```python
from build123d import *

# Parameters (mm, degrees)
CROQUIS1_R              = 5
CROQUIS1_R_2            = 3.25
SALIENTE_EXTRUIR1_DEPTH = 1
CORTAR_EXTRUIR1_DEPTH   = 10


with BuildPart() as part:
    # Croquis1 → Saliente-Extruir1 (new body)
    with BuildSketch(Plane.XY):
        Circle(CROQUIS1_R)
        Circle(CROQUIS1_R_2, mode=Mode.SUBTRACT)
    extrude(amount=SALIENTE_EXTRUIR1_DEPTH)

    # Croquis2 → Cortar-Extruir1 (cut)
    with BuildSketch(Plane.XY.offset(1)):
        Polygon((-2.6, -3), (-3.274652692, -3.778445414), (-3.274652692, -6), (-2.6, -6), (2.6, -6), (3.274652692, -6), (3.274652692, -3.778445414), (2.6, -3), (2.6, 0), (-2.6, 0), align=None)
    extrude(amount=-CORTAR_EXTRUIR1_DEPTH, mode=Mode.SUBTRACT)


solid = part.part
```
For this review, take the finished solid that the model builds, in its own axes (mm). A direction names the side the tool comes from. Coordinates: 2 decimals unless noted, no trailing zeros. Loops run counter-clockwise (first coordinate to the right, second up) from the corner with the lowest first, then second, coordinate; pieces in that order, holes last. Notation, with made-up numbers: (-35.75, 73.5) - (-8.75, 73.5) arc R16 cw to (-8.75, 94.5) - close; hole circle Ø1 at (-3.5, 12.5). An arc over 180 degrees is marked (long way). Use one line per item in the form item = value. Start each with the question number.
1) Draft analysis for pull direction X (two halves, no side actions). For faces 1 (the face through (0.17, 4.997, 0.493)), 2 (the face through (0.1, 3.25, 0.49)), 3 (the face through (2.6, -2.5, 0.5)), 4 (the face through (0, 4, 0)), state which applies: released by +X, released by -X, zero draft, split by the parting line, or undercut.
2) Take a section at B-B (z = 0.15). State the section outline as (x, y) points.
3) Take a section at A-A (y = 0). State the section outline as (x, z) points.
4) To check wall thickness, follow probe 1 along X at (y, z) = (0, 0.3); probe 2 along Y at (x, z) = (0, 0.65); probe 3 along X at (y, z) = (2.25, 0.35). State the ranges of each line that lie inside material, in increasing order. Write a range as from..to.
5) Take a section at C-C (x = -3). State the section outline as (y, z) points, plus the area to 3 significant figures.
6) Take a section at D-D (x = 0). State the section outline as (y, z) points.
7) For faces 5 (the face through (0, 4, 1)), 6 (the face through (-2.6, -2.5, 0.5)), list the 3-axis set-ups (+Z, -Z, +X, -X, +Y, -Y) from which the entire face can be reached by the end or side of a thin tool; tool diameter is ignored.
From the geometry:
q1.face_1 = split by the parting line
q1.face_2 = undercut
q1.face_3 = undercut
q1.face_4 = zero draft
q2.outline = (-3.27, -3.78) - (-2.6, -3) - (-2.6, -1.95) arc R3.25 cw (long way) to (2.6, -1.95) - (2.6, -3) - (3.27, -3.78) arc R5 ccw (long way) to start
q3.outline = (-5, 0) - (-3.25, 0) - (-3.25, 1) - (-5, 1) - close; (3.25, 0) - (5, 0) - (5, 1) - (3.25, 1) - close
q4.probe_1 = -5..-3.25, 3.25..5
q4.probe_2 = 3.25..5
q4.probe_3 = -4.47..-2.35, 2.35..4.47
q5.outline = (-3.46, 0) - (-1.25, 0) - (-1.25, 1) - (-3.46, 1) - close; (1.25, 0) - (4, 0) - (4, 1) - (1.25, 1) - close
q5.area = 4.96 mm2
q6.outline = (3.25, 0) - (5, 0) - (5, 1) - (3.25, 1) - close
q7.face_5 = +Z, +X, -X, +Y, -Y
q7.face_6 = +Z, -Z, -Y
